from build123d import *

# Parameters (mm, degrees)
F0_R     = 44.45
F1_DEPTH = 3.81
F2_R     = 10.16
F3_DEPTH = 76.2
F5_DEPTH = 10.8966


with BuildPart() as f1:
    # F0 (on Front) → F1 (new body)
    with BuildSketch(Plane.XZ):
        Circle(F0_R)
        with BuildLine():
            ThreePointArc((7.631228, 40.563407), (29.185832, 29.185832), (40.563407, 7.631228))
            ThreePointArc((40.563407, 7.631228), (41.096717, 3.832167), (41.275, 0))
            ThreePointArc((41.275, 0), (41.096717, -3.832167), (40.563407, -7.631228))
            ThreePointArc((40.563407, -7.631228), (29.185832, -29.185832), (7.631228, -40.563407))
            ThreePointArc((7.631228, -40.563407), (0, -41.275), (-7.631228, -40.563407))
            ThreePointArc((-7.631228, -40.563407), (-29.185832, -29.185832), (-40.563407, -7.631228))
            ThreePointArc((-40.563407, -7.631228), (-41.275, 0), (-40.563407, 7.631228))
            ThreePointArc((-40.563407, 7.631228), (-29.185832, 29.185832), (-7.631228, 40.563407))
            ThreePointArc((-7.631228, 40.563407), (0, 41.275), (7.631228, 40.563407))
        make_face(mode=Mode.SUBTRACT)
        with BuildLine():
            ThreePointArc((-17.454709, -7.631228), (-19.05, 0), (-17.454709, 7.631228))
            Line((-17.454709, 7.631228), (-40.563407, 7.631228))
            Line((-40.563407, 7.631228), (-40.563407, -7.631228))
            Line((-40.563407, -7.631228), (-17.454709, -7.631228))
        make_face()
        with BuildLine():
            Line((17.454709, -7.631228), (17.454709, 7.631228))
            ThreePointArc((17.454709, 7.631228), (13.470384, 13.470384), (7.631228, 17.454709))
            Line((7.631228, 17.454709), (-7.631228, 17.454709))
            ThreePointArc((-7.631228, 17.454709), (-13.470384, 13.470384), (-17.454709, 7.631228))
            Line((-17.454709, 7.631228), (-17.454709, -7.631228))
            ThreePointArc((-17.454709, -7.631228), (-13.470384, -13.470384), (-7.631228, -17.454709))
            Line((-7.631228, -17.454709), (7.631228, -17.454709))
            ThreePointArc((7.631228, -17.454709), (13.470384, -13.470384), (17.454709, -7.631228))
        make_face()
        with BuildLine():
            Line((-17.454709, -7.631228), (-17.454709, 7.631228))
            ThreePointArc((-17.454709, 7.631228), (-19.05, 0), (-17.454709, -7.631228))
        make_face()
        with BuildLine():
            Line((-7.631228, 17.454709), (7.631228, 17.454709))
            ThreePointArc((7.631228, 17.454709), (0, 19.05), (-7.631228, 17.454709))
        make_face()
        with BuildLine():
            ThreePointArc((17.454709, -7.631228), (18.646913, -3.898096), (19.05, 0))
            ThreePointArc((19.05, 0), (18.646913, 3.898096), (17.454709, 7.631228))
            Line((17.454709, 7.631228), (17.454709, -7.631228))
        make_face()
        with BuildLine():
            ThreePointArc((41.275, 0), (41.096717, 3.832167), (40.563407, 7.631228))
            Line((40.563407, 7.631228), (40.563407, -7.631228))
            ThreePointArc((40.563407, -7.631228), (41.096717, -3.832167), (41.275, 0))
        make_face()
        with BuildLine():
            ThreePointArc((17.454709, 7.631228), (18.646913, 3.898096), (19.05, 0))
            ThreePointArc((19.05, 0), (18.646913, -3.898096), (17.454709, -7.631228))
            Line((17.454709, -7.631228), (40.563407, -7.631228))
            Line((40.563407, -7.631228), (40.563407, 7.631228))
            Line((40.563407, 7.631228), (17.454709, 7.631228))
        make_face()
        with BuildLine():
            Line((7.631228, -40.563407), (7.631228, -17.454709))
            ThreePointArc((7.631228, -17.454709), (0, -19.05), (-7.631228, -17.454709))
            Line((-7.631228, -17.454709), (-7.631228, -40.563407))
            Line((-7.631228, -40.563407), (7.631228, -40.563407))
        make_face()
        with BuildLine():
            ThreePointArc((-7.631228, -17.454709), (0, -19.05), (7.631228, -17.454709))
            Line((7.631228, -17.454709), (-7.631228, -17.454709))
        make_face()
        with BuildLine():
            ThreePointArc((-7.631228, -40.563407), (0, -41.275), (7.631228, -40.563407))
            Line((7.631228, -40.563407), (-7.631228, -40.563407))
        make_face()
        with BuildLine():
            Line((-40.563407, -7.631228), (-40.563407, 7.631228))
            ThreePointArc((-40.563407, 7.631228), (-41.275, 0), (-40.563407, -7.631228))
        make_face()
        with BuildLine():
            ThreePointArc((-7.631228, 17.454709), (0, 19.05), (7.631228, 17.454709))
            Line((7.631228, 17.454709), (7.631228, 40.563407))
            Line((7.631228, 40.563407), (-7.631228, 40.563407))
            Line((-7.631228, 40.563407), (-7.631228, 17.454709))
        make_face()
        with BuildLine():
            Line((-7.631228, 40.563407), (7.631228, 40.563407))
            ThreePointArc((7.631228, 40.563407), (0, 41.275), (-7.631228, 40.563407))
        make_face()
    extrude(amount=F1_DEPTH)

    # F2 (on face) → F3 (join)
    with BuildSketch(Plane.XZ.offset(3.81)):
        Circle(F2_R)
    extrude(amount=F3_DEPTH)

    # F4 (on face) → F5 (join)
    with BuildSketch(Plane.XZ.offset(80.01)):
        Polygon((3.102705, 9.00549), (-7.605941, 5.733697), (-7.803435, -5.46187), (2.783154, -9.109318), (9.523518, -0.167998), align=None)
    extrude(amount=F5_DEPTH)


solid = f1.part
Part model, mm, in its own coordinate system. A direction names the side the tool comes from. Coordinates: 2 decimals unless noted, no trailing zeros. Order: outer loops, then holes, each group sorted by start corner. A loop starts at its lowest first (then second) coordinate and runs counter-clockwise, first axis right, second up.
(1) Slice it at D-D, the plane z = 3.5. Write the cut outline in (x, y).
Check sheet entries:
outline: (-44.31, -3.81) - (-9.54, -3.81) - (-9.54, -80.01) - (-7.65, -80.01) - (-7.65, -90.91) - (6.96, -90.91) - (6.96, -80.01) - (9.54, -80.01) - (9.54, -3.81) - (44.31, -3.81) - (44.31, 0) - (-44.31, 0) - close
(2) Probe L1, parallel to Y at x = -1, z = 16; L2, parallel to Y at x = -4.5, z = 7.5; L3, parallel to Z at x = 3, y = -27. List the from-to ranges inside material, lowest first.
Check sheet entries:
L1: y = -3.81 to 0
L2: y = -80.01 to 0
L3: z = -9.71 to 9.71
(3) Slice it at B-B, the plane x = 31. Write the cut outline in (y, z), and give its area (3 significant figures).
Check sheet entries:
outline: (-3.81, -31.86) - (0, -31.86) - (0, -27.25) - (-3.81, -27.25) - close; (-3.81, -7.63) - (0, -7.63) - (0, 7.63) - (-3.81, 7.63) - close; (-3.81, 27.25) - (0, 27.25) - (0, 31.86) - (-3.81, 31.86) - close
area: 93.2 mm2
(4) Pin check, flat tips, straight feed: pin 1 Ø1 at (x, z) = (-6, -28.5) entering from -Y; pin 2 Ø1.9 at (y, z) = (-2, 26) entering from -X; pin 3 Ø4 at (x, y) = (29, -1.5) entering from -Z. Stop position of each tip, or through.
Check sheet entries:
pin 1: stops at y = -3.81
pin 2: stops at x = -36.72
pin 3: stops at z = -35.31
(5) Slice it at A-A, the plane z = -29. Write the cut outline in (x, y).
Check sheet entries:
outline: (-33.69, -3.81) - (-29.37, -3.81) - (-29.37, 0) - (-33.69, 0) - close; (-7.63, -3.81) - (7.63, -3.81) - (7.63, 0) - (-7.63, 0) - close; (29.37, -3.81) - (33.69, -3.81) - (33.69, 0) - (29.37, 0) - close
(6) Pull direction Z, two halves, no side cores. Call faces 1 (the face through (29, -2, -7.631)), 2 (the face through (1, -90.907, 0)), 3 (the face through (6.106, -85.382, -4.701)): pulls with the +Z half, pulls with the -Z half, needs draft (parallel to the pull), parting line crosses it, or undercut.
Check sheet entries:
face 1: undercut
face 2: needs draft
face 3: pulls with the -Z half
(7) Tool access for faces 4 (the face through (-2.18, -85.38, 7.39)), 5 (the face through (13.4, -1.88, -13.54)), 6 (the face through (-1, 0, 1)), 7 (the face through (-10, -3.81, -3)): list every direction of +Z, -Z, +X, -X, +Y, -Y with a clear straight run to the whole face (end or side of a thin tool).
Check sheet entries:
face 4: +Z, -X, -Y
face 5: +Y, -Y
face 6: +Z, -Z, +X, -X, +Y
face 7: -Y
(8) Slice it at C-C, the plane y = -81.5. Write the cut outline in (x, z), and give its area (3 significant figures).
Check sheet entries:
outline: (-7.8, -5.46) - (2.78, -9.11) - (9.52, -0.17) - (3.1, 9.01) - (-7.61, 5.73) - close
area: 216 mm2
